Input: part model. Units: mm. Frame: model coordinates. A direction names the side the tool comes from. Give positions to 0.01 mm unless a question says otherwise; leave off trailing zeros. Loops run counter-clockwise (first coordinate to the right, second up) from the corner with the lowest first, then second, coordinate; pieces in that order, holes last. Notation, with made-up numbers: (40, -6.5) - (79, -6.5) arc R25 cw to (79, 12.5) - close; hole circle Ø3 at (72, -14.5). An arc over 180 degrees is marked (long way). Answer as a JSON object with one key per item and string values.
Autodesk Inventor part; units mm, degrees
ref_plane "YZ Plane" through (0, 0, 0) normal (1, 0, 0) x (0, 1, 0)
ref_plane "XZ Plane" through (0, 0, 0) normal (0, 1, 0) x (-1, 0, 0)
ref_plane "XY Plane" through (0, 0, 0) normal (0, 0, 1) x (1, 0, 0)
sketch "Эскиз1" plane through (0, 0, 0) normal (1, 0, 0) x (0, 1, 0)
  circle A0 centre (35.2311, -22.6062) radius 9.3
  circle A1 centre (0, -38.8201) radius 6.1 construction
  circle A2 centre (0, 0) radius 4.85 construction
  circle A3 centre (35.8147, -49.5529) radius 3.55
  line L0 (6.0968, -38.6237) -> (4.8475, 0.1562) construction
  line L1 (-4.8475, 0.1562) -> (-6.0968, -38.6237) construction
  line L2 (0, 0) -> (0, -38.8201) construction
  circle A4 centre (0, -38.8201) radius 4.1
  circle A5 centre (0, 0) radius 2.5
  circle A6 centre (0, -38.8201) radius 15 construction
  circle A7 centre (0, 0) radius 14 construction
  circle A8 centre (0, -38.8201) radius 7.6
  circle A9 centre (0, 0) radius 7 construction
  line L3 (7.5465, -39.7207) -> (12.114, -1.4456)
  line L4 (-7.5465, -39.7207) -> (-12.114, -1.4456)
  circle A10 centre (0, 0) radius 8.8 construction
  circle A11 centre (0, 0) radius 12.2
  circle A12 centre (6.8983, -19.8347) radius 1.6
  circle A13 centre (-7.3019, -16.4524) radius 1.6
  point P0 (-7, 0)
  point P1 (-7.5465, -39.7207)
  point P2 (-12.114, -1.4456)
  dimension "d0" = 18.6
  dimension "d1" = 12.2
  dimension "d2" = 9.7
  dimension "d3" = 7.1
  dimension "d8" = 38.8201
  dimension "d13" = 38.8
  dimension "d14" = 38.8
  dimension "d23" = 8.2
  dimension "d24" = 5
  dimension "d25" = 30
  dimension "d26" = 28
  dimension "d28" = 14
  dimension "d31" = 17.6
  dimension "d32" = 3.4
  dimension "d56" = 3.5
  dimension "d58" = 3.2
  dimension "d59" = 3
  dimension "d60" = 21
  dimension "d61" = 3.2
  dimension "d62" = 3
  dimension "d63" = 18
extrude "Выдавливание4" add sketch "Эскиз1" along normal blind 3 contours A8 | A8 L4 A11 L3 | A11
sketch "Эскиз4" plane through (0, 0, 0) normal (-1, 0, 0) x (0, 0, 1)
  circle A0 centre (-38.8201, 0) radius 4.1 construction
  arc A1 (-1.4456, -12.114) -> (-1.4456, 12.114) centre (0, 0) ccw construction
  line L0 (-39.7207, 7.5465) -> (-1.4456, 12.114) construction
  arc A2 (-39.7207, 7.5465) -> (-39.7207, -7.5465) centre (-38.8201, 0) ccw construction
  line L1 (-1.4456, -12.114) -> (-39.7207, -7.5465) construction
  line L2 (0, 0) -> (0, 12.2) construction
  arc A3 (-1.4456, -12.114) -> (-1.4456, 12.114) centre (0, 0) ccw construction
  line L3 (0, 0) -> (12.2, 0) construction
  circle A4 centre (5.6569, 5.6569) radius 1.7
  line L4 (5.6569, 5.6569) -> (0, 0) construction
  circle A5 centre (-6.364, 6.364) radius 1.7
  line L5 (0, 0) -> (-6.364, 6.364) construction
  circle A6 centre (-5.6569, -5.6569) radius 1.7
  circle A7 centre (6.364, -6.364) radius 1.7
  dimension "d65" = 45
  dimension "d66" = 3.4
  dimension "d67" = 3.4
  dimension "d68" = 45
  dimension "d69" = 16
  dimension "d70" = 18
extrude "Выдавливание5" cut sketch "Эскиз4" against normal blind 3
sketch "Эскиз5" plane through (3, 0, 0) normal (1, 0, 0) x (0, 0, -1)
  circle A0 centre (0, 0) radius 3.75
  dimension "d38" = 7.5
extrude "Выдавливание6" cut sketch "Эскиз5" against normal blind 3
sketch "Эскиз6" plane through (3, 0, 0) normal (1, 0, 0) x (0, 0, -1)
  circle A0 centre (0, -18) radius 2
  circle A1 centre (0, 0) radius 3.75 construction
  circle A2 centre (-5.6569, 5.6569) radius 1.7 construction
  circle A3 centre (38.8201, 0) radius 4.1 construction
  line L0 (39.7207, 7.5465) -> (1.4456, 12.114) construction
  arc A4 (1.4456, 12.114) -> (1.4456, -12.114) centre (0, 0) ccw construction
  line L1 (1.4456, -12.114) -> (39.7207, -7.5465) construction
  arc A5 (39.7207, -7.5465) -> (39.7207, 7.5465) centre (38.8201, 0) ccw construction
  line L2 (0, 0) -> (0, -26.6004) construction
  circle A6 centre (0, 0) radius 14 construction
  line L3 (-10.8605, -5.5578) -> (-3.5608, -19.8222)
  arc A7 (0, -14) -> (-3.5608, -19.8222) centre (0, -18) ccw construction
  line L4 (2.8284, -20.8284) -> (12.911, -10.7458)
  line L5 (1.4456, -12.114) -> (39.7207, -7.5465) construction
  arc A8 (2.8284, -20.8284) -> (0, -14) centre (0, -18) ccw construction
  arc A9 (-3.5608, -19.8222) -> (2.8284, -20.8284) centre (0, -18) ccw
  line L6 (-10.8605, -5.5578) -> (-10.1465, -5.5578)
  line L7 (-10.1465, -5.5578) -> (-6.8136, -9.4237)
  line L8 (-6.8136, -9.4237) -> (5.1237, -10.512)
  line L9 (5.1237, -10.512) -> (12.911, -10.7458)
  dimension "d42" = 28
  dimension "d41" = 4
  dimension "d43" = 18
  dimension "d44" = 8
  dimension "d45" = 45
extrude "Выдавливание7" [suppressed]
sketch "Эскиз7" plane through (3, 0, 0) normal (1, 0, 0) x (0, 0, -1)
  line L0 (0, 0) -> (0, -29.4139) construction
  circle A0 centre (-9, -15.5885) radius 2.75
  line L1 (-9, -15.5885) -> (0, 0) construction
  circle A1 centre (0, 0) radius 14 construction
  circle A2 centre (0, 0) radius 18 construction
  arc A3 (-5.7, -21.3042) -> (-15.4588, -14.2305) centre (-9, -15.5885) ccw construction
  circle A4 centre (0, 0) radius 3.75 construction
  circle A5 centre (-5.6569, 5.6569) radius 1.7 construction
  circle A6 centre (38.8201, 0) radius 4.1 construction
  line L2 (39.7207, 7.5465) -> (1.4456, 12.114) construction
  arc A7 (1.4456, 12.114) -> (1.4456, -12.114) centre (0, 0) ccw
  line L3 (1.4456, -12.114) -> (39.7207, -7.5465)
  arc A8 (39.7207, -7.5465) -> (39.7207, 7.5465) centre (38.8201, 0) ccw construction
  line L4 (-11.939, 2.5102) -> (-15.4588, -14.2305)
  line L5 (-5.7, -21.3042) -> (12.5035, -10.7945)
  line L6 (1.4456, -12.114) -> (39.7207, -7.5465) construction
  arc A9 (-15.4588, -14.2305) -> (-5.7, -21.3042) centre (-9, -15.5885) ccw
  circle A10 centre (-9, -15.5885) radius 4.1
  point P0 (12.5035, -10.7945)
  dimension "d48" = 5.5
  dimension "d49" = 330
  dimension "d50" = 28
  dimension "d51" = 4
  dimension "d53" = 30
  dimension "d71" = 8.2
  dimension "d76" = 2.5
extrude "Выдавливание8" add sketch "Эскиз7" against normal up to surface (3 mm away) contours A7 L3 L5 A9 L4 | A10
extrude "Выдавливание9" cut sketch "Эскиз7" against normal blind 3 contours A10
extrude "Выдавливание10" add sketch "Эскиз7" against normal blind 0.7 contours A10
properties part number "_3DПЕЧАТЬ"
Item 1: Material intervals for line 1 (Z direction, x = 2.3, y = -6); line 2 (Z direction, x = 2.1, y = 2.5); line 3 (Z direction, x = 1.5, y = -7), sorted ascending. Write a range as [from, to].
Geometry check:
{"line 1": "z = [-43.48, -17.38], [-15.52, -7.32], [-3.99, 4.7], [8.02, 13.73]", "line 2": "z = [-46, -42.07], [-35.57, -2.8], [2.8, 11.94]", "line 3": "z = [-41.78, -18.02], [-14.88, -6.7], [-4.61, 4.79], [7.94, 13.94]"}
Item 2: Contact query for flat-ended pins moving along their axis: P1, Ø1.5, axis at x = 2, z = -18.5, coming from the -Y side; P2, Ø6.5, axis at y = 0, z = -38.82, coming from the -X side; P3, Ø5.5, axis at y = 6.364, z = -6.364, coming from the -X side; P4, Ø1, axis at x = 1, y = -6.5, coming from the -Z side. Output: stop coordinate, or through.
Geometry check:
{"P1": "stops at y = -10.17", "P2": "passes through", "P3": "stops at x = 0", "P4": "stops at z = -43.48"}
Item 3: Cut plane B-B (z = 0). Return loops of the section in (x, y).
Geometry check:
{"outline": "(0, -18.01) - (3, -18.01) - (3, -3.75) - (0, -3.75) - close; (0, 3.75) - (3, 3.75) - (3, 12.2) - (0, 12.2) - close"}
Item 4: Mould query, pull axis Z, two halves, no side actions, for faces 3 (the face through (1.521, -16.123, -3.274)), 4 (the face through (1.48, 5.01, 7.23)), 5 (the face through (1.521, -5.743, 13.674)). Classes: released by +Z, released by -Z, zero draft, split by the parting line, or undercut.
Geometry check:
{"face 3": "released by -Z", "face 4": "undercut", "face 5": "released by +Z"}
Item 5: Cut plane D-D (x = 0.8). Give the number of separate pieces and of enclosed holes in the cut face, then the cut area to 3 significant figures.
Geometry check:
{"separate pieces": "1", "enclosed holes": "9", "area": "1,110 mm2"}
Item 6: Cut plane C-C (y = 0). Return loops of the section in (x, z).
Geometry check:
{"outline": "(0, -46.42) - (3, -46.42) - (3, -42.92) - (0, -42.92) - close; (0, -34.72) - (3, -34.72) - (3, -3.75) - (0, -3.75) - close; (0, 3.75) - (3, 3.75) - (3, 12.47) - (0, 12.47) - close"}
Item 7: Cut plane A-A (y = -17.5). Return loops of the section in (x, z).
Geometry check:
{"outline": "(0, -0.89) - (3, -0.89) - (3, 7.02) - (2.3, 7.02) - (2.3, 5.37) - (0, 5.37) - close; (0, 12.63) - (2.3, 12.63) - (2.3, 10.98) - (3, 10.98) - (3, 15.32) - (0, 15.32) - close"}
Item 8: Access query for faces 1 (the face through (2.3, -16, 6)), 2 (the face through (1.479, -7.316, -6.025)). Directions: +Z, -Z, +X, -X, +Y, -Y. A direction counts if a zero-diameter tool reaches every point of the face in a straight line with its end or side. Return the directions, or none.
Geometry check:
{"face 1": "-X", "face 2": "+X, -X"}
